from build123d import *

# Parameters (mm, degrees)
F1_DEPTH = 47.625
F2_R     = 6.35
F3_DEPTH = 47.625
F4_R     = 15.875
F4_R_2   = 6.35
F5_DEPTH = 15.875


with BuildPart() as f1:
    # F0 (on Front) → F1 (new body)
    with BuildSketch(Plane.XZ):
        with BuildLine():
            ThreePointArc((-104.775, 63.5), (-136.525, 31.75), (-104.775, 0))
            Line((-104.775, 0), (-104.775, 63.5))
        make_face()
        with BuildLine():
            Line((-104.775, 0), (0, 0))
            Line((0, 0), (0, 31.75))
            ThreePointArc((0, 31.75), (-12.457359, 34.295947), (-22.916874, 41.525483))
            ThreePointArc((-22.916874, 41.525483), (-29.459067, 51.658299), (-31.75, 63.5))
            Line((-31.75, 63.5), (-104.775, 63.5))
            Line((-104.775, 63.5), (-104.775, 0))
        make_face()
    extrude(amount=F1_DEPTH)

    # F2 (on face) → F3 (cut)
    with BuildSketch(Plane.XZ.offset(47.625)):
        with Locations((-104.775, 31.75)):
            Circle(F2_R)
    extrude(amount=-F3_DEPTH, mode=Mode.SUBTRACT)

    # F4 (on face) → F5 (cut)
    with BuildSketch(Plane.XZ.offset(47.625)):
        with Locations((-104.775, 31.75)):
            Circle(F4_R)
        with Locations((-104.775, 31.75)):
            Circle(F4_R_2, mode=Mode.SUBTRACT)
    extrude(amount=-F5_DEPTH, mode=Mode.SUBTRACT)


solid = f1.part
Read the model definition and answer for the solid it produces. Units are mm, in the model's axes. A direction names the side the tool comes from. Give positions to 0.01 mm unless a question says otherwise; leave off trailing zeros. Write each loop counter-clockwise with the first axis right and the second up, starting at its lowest first coordinate (ties: lowest second). Pieces come first, ordered by that corner, then holes. Notation, with made-up numbers: M 21,6.5 L 77,6.5 A34 ccw 77,45.5 Z; hole C 18.5,9 d6. An arc over 180 degrees is marked long. One line per item, written item: value. Start each with the question number.
(1) Find section C-C (z = 28.5). Determine the outline of the cut face in (x, y) (3 decimals).
(2) Determine the mould class of faces 3 (the flat face through (-69, -47.625, 32)), 4 (the flat face through (-68, -23, 63.5)), 5 (the cylindrical face through (-98.72, -16.1, 33.66)), 6 (the flat face through (-53, -23, 0)) for opening direction Z: pulls with the +Z half, pulls with the -Z half, needs draft (parallel to the pull), parting line crosses it, or undercut.
(3) Find the intervals of material crossed by line 1 (X direction, y = -39, z = 31); line 2 (X direction, y = -32, z = 40); line 3 (Z direction, x = -23, y = -16), in increasing order.
(4) Find section A-A (y = -11.5). Determine the outline of the cut face in (x, z) (3 decimals), plus the area to 3 significant figures.
(5) A tool of negligible diameter and unlimited length cuts with its end or side. For faces 1 (the flat face through (-69, 0, 32)), 2 (the cylindrical face through (-120.635, -39.799, 32.448)), from which of +Z, -Z, +X, -X, +Y, -Y can it reach the whole face along a straight path? Write none if from no direction.
(6) Find section D-D (x = -10). Determine the outline of the cut face in (y, z) (3 decimals).
(7) Flat-ended cylindrical pins translate along their axes: pin 1 Ø1 at (x, z) = (-111, 36.5) entering from +Y; pin 2 Ø5 at (y, z) = (-41, 42.5) entering from -X; pin 3 Ø5 at (y, z) = (-20.5, 38) entering from +X. Find the tip coordinate at first contact, or state that the pin passes through.
(8) Find section B-B (x = -100). Determine the outline of the cut face in (y, z) (3 decimals).
Results below:
1. outline: M -136.358,-47.625 L -120.314,-47.625 L -120.314,-31.75 L -110.23,-31.75 L -110.23,0 L -136.358,0 Z; M -99.32,-31.75 L -89.236,-31.75 L -89.236,-47.625 L 0,-47.625 L 0,0 L -99.32,0 Z
2. face 3: needs draft
2. face 4: pulls with the +Z half
2. face 5: undercut
2. face 6: pulls with the -Z half
3. line 1: x = -136.52 to -120.63, -88.92 to 0
3. line 2: x = -135.43 to -118.34, -91.21 to -21.35
3. line 3: z = 0 to 41.61
4. outline: M -104.775,0 L 0,0 L 0,31.75 A31.75 cw -22.917,41.525 A31.75 cw -31.75,63.5 L -104.775,63.5 A31.75 ccw Z; hole C -104.775,31.75 d12.7
4. area: 7,320 mm^2
5. face 1: +Z, -Z, +X, -X, +Y
5. face 2: -Y
6. outline: M -47.625,0 L 0,0 L 0,33.366 L -47.625,33.366 Z
7. pin 1: stops at y = 0
7. pin 2: stops at x = -135.43
7. pin 3: stops at x = -14.97
8. outline: M -47.625,0 L 0,0 L 0,27.564 L -31.75,27.564 L -31.75,16.61 L -47.625,16.61 Z; M -47.625,46.89 L -31.75,46.89 L -31.75,35.936 L 0,35.936 L 0,63.5 L -47.625,63.5 Z
